Geometry check sheet. Reference: the model listing, model coordinates, mm. Face numbers are marked on the shaded views. A direction names the side the tool comes from. Round coordinates to 2 decimals unless told otherwise and drop trailing zeros. Order: outer loops, then holes, each group sorted by start corner. A loop starts at its lowest first (then second) coordinate and runs counter-clockwise, first axis right, second up. Notation, with made-up numbers: (-11.75, 60.25) -> (2.25, 60.25) arc R16 cw to (2.25, 89.25) -> close; hole circle Ø8 at (40, -37.75). An arc over 180 degrees is marked (long way). Use a Markdown table: item, result. Add a question column.
Item 1: Material ranges on probe 1 along X at (y, z) = (-23.2, 0); probe 2 along Z at (x, y) = (20.25, 0); probe 3 along Y at (x, z) = (12, 0), recorded low to high. Write a range as [from, to].
Item 2: Sectioned sample at B-B, the plane x = 25. Record the cut outline in (y, z), and give its area (3 significant figures).
Item 3: Set-up check for the marked faces 4 and 5: record each of +Z, -Z, +X, -X, +Y, -Y from which the full face is reachable in a straight line by a thin tool's end or side.
Item 4: Sectioned sample at C-C, the plane z = 16.5. Record the cut outline in (x, y).
Item 5: Sectioned sample at A-A, the plane z = 0. Record the cut outline in (x, y).
Item 6: Gauge pin test, flat ends, axial feed: pin 1 Ø5 at (x, y) = (1, 4) entering from -Z; pin 2 Ø0.9 at (x, z) = (-1.5, 2.5) entering from +Y; pin 3 Ø10 at (x, z) = (1.5, -11.5) entering from +Y. Record the tip position at first contact, or that the pin passes through.
Item 7: Sectioned sample at D-D, the plane x = 9. Record the cut outline in (y, z), and give its area (3 significant figures).
Item 8: Mould release check, pull along Z, two halves, no side actions. Record for the marked faces 1, 2 and 3: pulls with the +Z half, pulls with the -Z half, needs draft (parallel to the pull), parting line crosses it, or undercut.
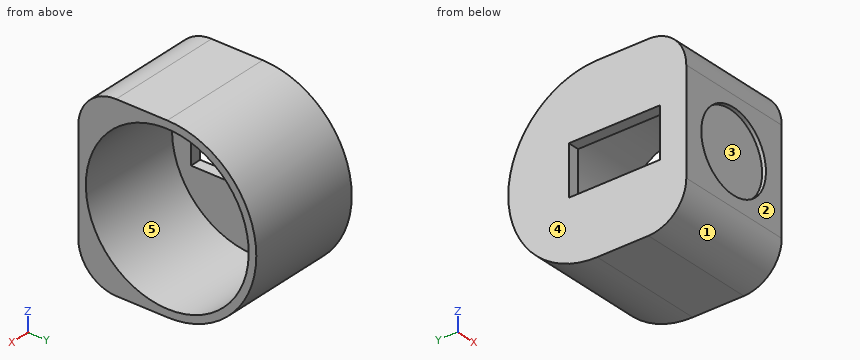
from build123d import *

# Parameters (mm, degrees)
SKETCH1_R           = 23.505813168
SKETCH1_R_2         = 21.505813168
BOSS_EXTRUDE1_DEPTH = 28
BOSS_EXTRUDE4_START = -3
SKETCH1_6_R         = 23.505813168
SKETCH1_6_R_2       = 21.505813168
SKETCH1_6_W         = 4
SKETCH1_6_H         = 13
BOSS_EXTRUDE4_DEPTH = 3
BOSS_EXTRUDE5_START = -31
BOSS_EXTRUDE5_DEPTH = 31
SKETCH3_R           = 10.5
CUT_EXTRUDE4_DEPTH  = 1


with BuildPart() as part:
    # Sketch1 → Boss-Extrude1 (new body)
    with BuildSketch(Plane.YZ):
        with Locations(Location((0, 0, 0), (0, 0, 270))):
            Circle(SKETCH1_R)
        with Locations(Location((0, 0, 0), (0, 0, 270))):
            Circle(SKETCH1_R_2, mode=Mode.SUBTRACT)
    extrude(amount=BOSS_EXTRUDE1_DEPTH)

    # Sketch1<6> → Boss-Extrude4 (add)
    # profile 1 of 5: a face of its own
    with BuildSketch(Plane.YZ.offset(BOSS_EXTRUDE4_START)):
        with Locations(Location((0, 0, 0), (0, 0, 270))):
            Circle(SKETCH1_6_R)
        with Locations(Location((0, 0, 0), (0, 0, 270))):
            Circle(SKETCH1_6_R_2, mode=Mode.SUBTRACT)
    # profile 2 of 5: a face of its own
    with BuildSketch(Plane.YZ.offset(BOSS_EXTRUDE4_START)):
        with BuildLine():
            Line((-20.5, -6.5), (-20.5, 6.5))
            ThreePointArc((-20.5, 6.5), (-21.505813168, 0), (-20.5, -6.5))
        make_face()
    # profile 3 of 5: a face of its own
    with BuildSketch(Plane.YZ.offset(BOSS_EXTRUDE4_START)):
        with Locations((-18.5, 0)):
            Rectangle(SKETCH1_6_W, SKETCH1_6_H)
    # profile 4 of 5: a face of its own
    with BuildSketch(Plane.YZ.offset(BOSS_EXTRUDE4_START)):
        with BuildLine():
            Line((-20.5, 6.5), (-16.5, 6.5))
            Line((-16.5, 6.5), (-7.925433742, 6.5))
            ThreePointArc((-7.925433742, 6.5), (3.451579649, 9.651378033), (10.25, 0))
            ThreePointArc((10.25, 0), (3.451579649, -9.651378033), (-7.925433742, -6.5))
            Line((-7.925433742, -6.5), (-16.5, -6.5))
            Line((-16.5, -6.5), (-20.5, -6.5))
            ThreePointArc((-20.5, -6.5), (3.288679831, -21.252872393), (21.505813168, 0))
            ThreePointArc((21.505813168, 0), (3.288679831, 21.252872393), (-20.5, 6.5))
        make_face()
    # profile 5 of 5: a face of its own
    with BuildSketch(Plane.YZ.offset(BOSS_EXTRUDE4_START)):
        with BuildLine():
            ThreePointArc((10.25, 0), (3.451579649, 9.651378033), (-7.925433742, 6.5))
            Line((-7.925433742, 6.5), (0, 6.5))
            Line((0, 6.5), (7.5, 6.5))
            Line((7.5, 6.5), (7.5, -6.5))
            Line((7.5, -6.5), (0, -6.5))
            Line((0, -6.5), (-7.925433742, -6.5))
            ThreePointArc((-7.925433742, -6.5), (3.451579649, -9.651378033), (10.25, 0))
        make_face()
    extrude(amount=BOSS_EXTRUDE4_DEPTH)

    # Sketch2 → Boss-Extrude5 (add)
    with BuildSketch(Plane.YZ.offset(28).offset(BOSS_EXTRUDE5_START)):
        with BuildLine():
            ThreePointArc((-23.505813168, 0), (-16.621119888, 16.621119888), (0, 23.505813168))
            Line((0, 23.505813168), (-13.505813168, 23.505813168))
            ThreePointArc((-13.505813168, 23.505813168), (-20.576880979, 20.576880979), (-23.505813168, 13.505813168))
            Line((-23.505813168, 13.505813168), (-23.505813168, 0))
        make_face()
        with BuildLine():
            ThreePointArc((0, -23.505813168), (-16.621119888, -16.621119888), (-23.505813168, 0))
            Line((-23.505813168, 0), (-23.505813168, -13.505813168))
            ThreePointArc((-23.505813168, -13.505813168), (-20.576880979, -20.576880979), (-13.505813168, -23.505813168))
            Line((-13.505813168, -23.505813168), (0, -23.505813168))
        make_face()
    extrude(amount=BOSS_EXTRUDE5_DEPTH)

    # Sketch3 → Cut-Extrude4 (cut)
    with BuildSketch(Plane.XZ.offset(23.505813168)):
        with Locations(Location((12.372081248, 0, 0), (0, 0, 270))):
            Circle(SKETCH3_R)
    extrude(amount=-CUT_EXTRUDE4_DEPTH, mode=Mode.SUBTRACT)


solid = part.part
Found:
| question | item | result |
|---|---|---|
| 1 | probe 1 | x = [-3, 1.87], [22.87, 28] |
| 1 | probe 2 | z = [-23.51, -21.51], [21.51, 23.51] |
| 1 | probe 3 | y = [-22.51, -21.51], [21.51, 23.51] |
| 2 | outline | (-23.51, -13.51) arc R10 ccw to (-13.51, -23.51) -> (0, -23.51) arc R23.51 ccw to (0, 23.51) -> (-13.51, 23.51) arc R10 ccw to (-23.51, 13.51) -> close; hole circle Ø43.01 at (0, 0) |
| 2 | area | 477 mm2 |
| 3 | face 4 | +Z, -Z, -X, +Y, -Y |
| 3 | face 5 | +X |
| 4 | outline | (-3, -23.05) -> (28, -23.05) -> (28, -13.79) -> (0, -13.79) -> (0, 13.79) -> (28, 13.79) -> (28, 16.74) -> (-3, 16.74) -> close |
| 5 | outline | (-3, -23.51) -> (1.87, -23.51) -> (1.87, -22.51) -> (22.87, -22.51) -> (22.87, -23.51) -> (28, -23.51) -> (28, -21.51) -> (0, -21.51) -> (0, -16.5) -> (-3, -16.5) -> close; (-3, 7.5) -> (0, 7.5) -> (0, 21.51) -> (28, 21.51) -> (28, 23.51) -> (-3, 23.51) -> close |
| 6 | pin 1 | stops at z = -23.46 |
| 6 | pin 2 | stops at y = 23.42 |
| 6 | pin 3 | stops at y = 22.59 |
| 7 | outline | (-23.51, -13.51) arc R10 ccw to (-13.51, -23.51) -> (0, -23.51) arc R23.51 ccw to (0, 23.51) -> (-13.51, 23.51) arc R10 ccw to (-23.51, 13.51) -> (-23.51, 9.94) -> (-22.51, 9.94) -> (-22.51, -9.94) -> (-23.51, -9.94) -> close; hole circle Ø43.01 at (0, 0) |
| 7 | area | 457 mm2 |
| 8 | face 1 | pulls with the -Z half |
| 8 | face 2 | needs draft |
| 8 | face 3 | undercut |
